Geometry: final body of the model. Coordinates: model frame, mm. Coordinates: 2 decimals unless noted, no trailing zeros. Order: outer loops, then holes, each group sorted by start corner. A loop starts at its lowest first (then second) coordinate and runs counter-clockwise, first axis right, second up. Notation, with made-up numbers: M 1.25,80 L 50.25,80 A12 ccw 50.25,92 Z; hole C 82.25,-28 d4. An arc over 180 degrees is marked long. One line per question, with ' | ' between items.
from build123d import *

# Parameters (mm, degrees)
SKETCH1_W           = 101.6
SKETCH1_H           = 77.11
BOSS_EXTRUDE1_DEPTH = 6.35
SKETCH2_R           = 98.5502
CUT_EXTRUDE1_DEPTH  = 7.35
SKETCH3_R           = 3.302
CUT_EXTRUDE2_DEPTH  = 7.35


with BuildPart() as part:
    # Sketch1 → Boss-Extrude1 (new body)
    with BuildSketch(Plane.XY):
        with Locations((1.062427377, -30.694895509)):
            Rectangle(SKETCH1_W, SKETCH1_H)
    extrude(amount=BOSS_EXTRUDE1_DEPTH)

    # Sketch2 → Cut-Extrude1 (cut, through all)
    with BuildSketch(Plane.XY.offset(6.35)):
        with Locations((1.501142757, -153.515944306)):
            Circle(SKETCH2_R)
    extrude(amount=-CUT_EXTRUDE1_DEPTH, mode=Mode.SUBTRACT)

    # Sketch3 → Cut-Extrude2 (cut, through all)
    with BuildSketch(Plane.XY.offset(6.35)):
        with Locations((-41.318062251, 0)):
            Circle(SKETCH3_R)
        with Locations((-13.318062251, 0)):
            Circle(SKETCH3_R)
        with Locations((14.681937749, 0)):
            Circle(SKETCH3_R)
        with Locations((42.681937749, 0)):
            Circle(SKETCH3_R)
        with Locations((-41.318062251, -28)):
            Circle(SKETCH3_R)
        with Locations((42.681937749, -28)):
            Circle(SKETCH3_R)
    extrude(amount=-CUT_EXTRUDE2_DEPTH, mode=Mode.SUBTRACT)


solid = part.part
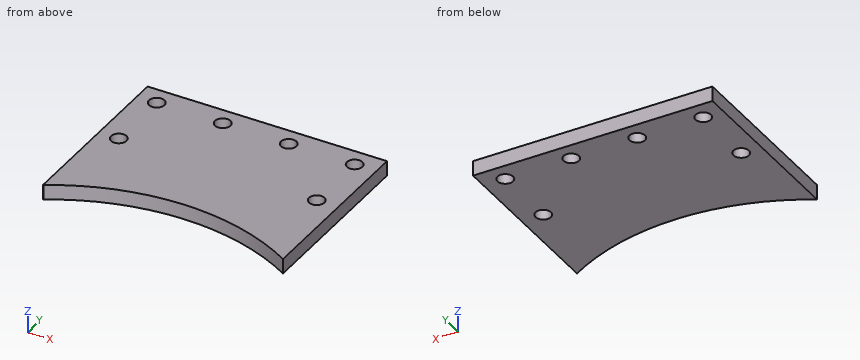
1. Section D-D, the plane x = 4.5. Output: boundary loops of the cut face in (y, z), and give its area (3 significant figures).
Response values:
outline: M -55.01,0 L 7.86,0 L 7.86,6.35 L -55.01,6.35 Z | area: 399 mm^2
2. Section A-A, the plane y = -28. Output: boundary loops of the cut face in (x, z), and give its area (3 significant figures).
Response values:
outline: M -49.74,0 L -44.62,0 L -44.62,6.35 L -49.74,6.35 Z; M -38.02,0 L 39.38,0 L 39.38,6.35 L -38.02,6.35 Z; M 45.98,0 L 51.86,0 L 51.86,6.35 L 45.98,6.35 Z | area: 561 mm^2
3. Section B-B, the plane y = 0. Output: boundary loops of the cut face in (x, z), and give its area (3 significant figures).
Response values:
outline: M -49.74,0 L -44.62,0 L -44.62,6.35 L -49.74,6.35 Z; M -38.02,0 L -16.62,0 L -16.62,6.35 L -38.02,6.35 Z; M -10.02,0 L 11.38,0 L 11.38,6.35 L -10.02,6.35 Z; M 17.98,0 L 39.38,0 L 39.38,6.35 L 17.98,6.35 Z; M 45.98,0 L 51.86,0 L 51.86,6.35 L 45.98,6.35 Z | area: 477 mm^2
4. Material intervals for line 1 (X direction, y = -1, z = 4) (3 decimals); line 2 (Y direction, x = 41, z = 0.5); line 3 (Y direction, x = 2, z = 2.5), sorted ascending. Write a range as [from, to].
Response values:
line 1: x = [-49.738, -44.465], [-38.171, -16.465], [-10.171, 11.535], [17.829, 39.535], [45.829, 51.862] | line 2: y = [-63.23, -30.84], [-25.16, -2.84], [2.84, 7.86] | line 3: y = [-54.97, 7.86]
5. Pin query (flat end, axial travel): P1, Ø6, axis at x = -41.32, y = -28, coming from the +Z side. Return the tip coordinate at first contact, or that it passes through.
Response values:
P1: passes through
6. Section C-C, the plane z = 1.5. Output: boundary loops of the cut face in (x, y), and give its area (3 significant figures).
Response values:
outline: M -49.74,-69.25 L -49.6,-69.25 A98.55 cw 51.86,-68.81 L 51.86,7.86 L -49.74,7.86 Z; hole C -41.32,-28 d6.6; hole C -41.32,0 d6.6; hole C -13.32,0 d6.6; hole C 14.68,0 d6.6; hole C 42.68,-28 d6.6; hole C 42.68,0 d6.6 | area: 6,640 mm^2
